```python
from build123d import *

# Parameters (mm, degrees)
ESQUISSE1_R        = 3.55
BOSS_EXTRU_1_DEPTH = 1


with BuildPart() as part:
    # Esquisse1 → Boss.-Extru.1 (new, symmetric)
    with BuildSketch(Plane.XY):
        Polygon((3.175426481, -5.5), (6.350852961, 0), (3.175426481, 5.5), (-3.175426481, 5.5), (-6.350852961, 0), (-3.175426481, -5.5), align=None)
        Circle(ESQUISSE1_R, mode=Mode.SUBTRACT)
    extrude(amount=BOSS_EXTRU_1_DEPTH, both=True)

    # Esquisse2 → Enlèvement de matière-Révolution1 (revolve, cut)
    with BuildSketch(Plane(origin=(0, 0, 0), x_dir=(1, 0, 0), z_dir=(0, 1, 0))):
        Polygon((-6.350852961, -0.4), (-5.450852961, -1), (-6.350852961, -1), align=None)
    enl_vement_de_mati_re_r_volution1 = revolve(axis=Axis((0, 0, -0.1), (0, 0, 1)), mode=Mode.SUBTRACT)

    # Symétrie2: Enlèvement de matière-Révolution1 across plane
    add(enl_vement_de_mati_re_r_volution1.mirror(Plane.XY), mode=Mode.SUBTRACT)


solid = part.part
```
Design review of the part built by this model. Coordinates are the model's own, in mm. Coordinates: 2 decimals unless noted, no trailing zeros. Loops run counter-clockwise (first coordinate to the right, second up) from the corner with the lowest first, then second, coordinate; pieces in that order, holes last. Notation, with made-up numbers: M 24.5,20.25 L 59.5,20.25 A17 ccw 59.5,34.25 Z; hole C -11,5 d3. An arc over 180 degrees is marked long. One line per question, with ' | ' between items.
(1) For pin 1 Ø1 at (y, z) = (2.5, 0.5) entering from +X; pin 2 Ø1 at (x, z) = (5, 0) entering from -Y, all flat-tipped, find the tip position at first contact; note any pin that passes through.
Filled in:
pin 1: stops at x = 5.2 | pin 2: stops at y = -3.21
(2) Wall thickness on probe 1 along Y at (x, z) = (0, 0.05); probe 2 along Y at (x, z) = (2.25, -0.05); probe 3 along X at (y, z) = (-0.5, -0.9): over which ranges is each line inside the solid? List them lowest first.
Filled in:
probe 1: y = -5.5 to -3.55, 3.55 to 5.5 | probe 2: y = -5.5 to -2.75, 2.75 to 5.5 | probe 3: x = -5.58 to -3.51, 3.51 to 5.58
(3) We need section C-C (z = 0.75). Give the boundary of the cut face in (x, y).
Filled in:
outline: M -5.72,-1.09 L -3.8,-4.41 A5.83 ccw -1.92,-5.5 L 1.92,-5.5 A5.83 ccw 3.8,-4.41 L 5.72,-1.09 A5.83 ccw 5.72,1.09 L 3.8,4.41 A5.83 ccw 1.92,5.5 L -1.92,5.5 A5.83 ccw -3.8,4.41 L -5.72,1.09 A5.83 ccw Z; hole C 0,0 d7.1
(4) We need section D-D (z = -0.55). Give the boundary of the cut face in (x, y).
Filled in:
outline: M -6.11,-0.41 L -3.41,-5.09 A6.13 ccw -2.7,-5.5 L 2.7,-5.5 A6.13 ccw 3.41,-5.09 L 6.11,-0.41 A6.13 ccw 6.11,0.41 L 3.41,5.09 A6.13 ccw 2.7,5.5 L -2.7,5.5 A6.13 ccw -3.41,5.09 L -6.11,0.41 A6.13 ccw Z; hole C 0,0 d7.1
(5) We need section A-A (z = 0.1). Give the boundary of the cut face in (x, y).
Filled in:
outline: M -6.35,0 L -3.18,-5.5 L 3.18,-5.5 L 6.35,0 L 3.18,5.5 L -3.18,5.5 Z; hole C 0,0 d7.1
(6) Draft analysis for pull direction Y (two halves, no side actions). For faces 1 (the face through (0, -4, 1)), 2 (the face through (4.74, -2.79, 0.01)), 3 (the face through (-0.46, 3.52, -0.01)), 4 (the face through (4.785, 2.712, 0.014)), state which applies: released by +Y, released by -Y, zero draft, split by the parting line, or undercut.
Filled in:
face 1: zero draft | face 2: released by -Y | face 3: undercut | face 4: released by +Y
(7) We need section B-B (x = 0). Give the boundary of the cut face in (y, z), and give its area (3 significant figures).
Filled in:
outline: M -5.5,-0.97 L -5.45,-1 L -3.55,-1 L -3.55,1 L -5.45,1 L -5.5,0.97 Z; M 3.55,-1 L 5.45,-1 L 5.5,-0.97 L 5.5,0.97 L 5.45,1 L 3.55,1 Z | area: 7.80 mm^2
